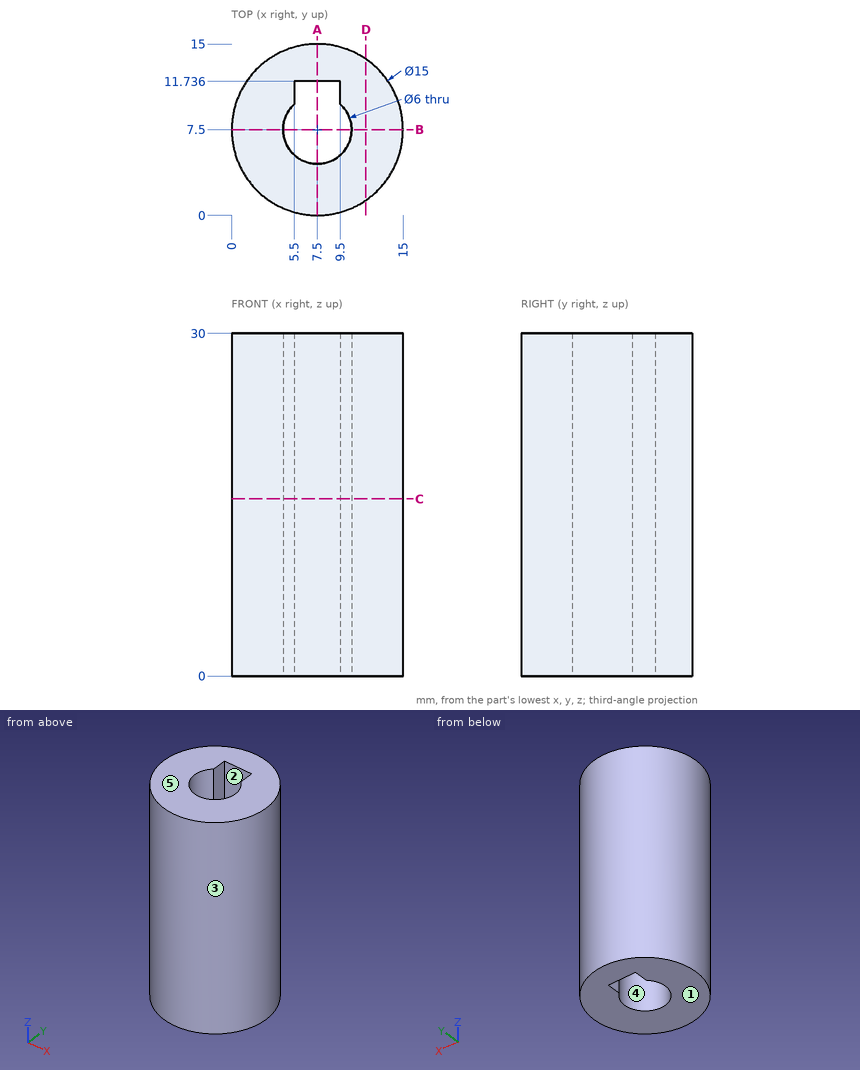
Could you check a few things on this drawing? It's one solid part, dimensions in mm from its lowest x, y, z. A direction names the side the tool comes from. Give positions to 0.01 mm unless a question says otherwise; leave off trailing zeros. Order: outer loops, then holes, each group sorted by start corner. A loop starts at its lowest first (then second) coordinate and runs counter-clockwise, first axis right, second up. Notation, with made-up numbers: (-26, 37) - (13, 37) arc R22 ccw to (13, 46) - close; hole circle Ø11 at (-14.75, 6.5). An arc over 180 degrees is marked (long way). Return JSON: item names as keys, results as strings. Group by question number.
Q1. Thinking about a two-plate mould opening in Y: for the marked faces 3, 4 and 5, which applies, pulls with the +Y half, pulls with the -Y half, needs draft (parallel to the pull), parting line crosses it, or undercut?
Q2. Suppose I cut it at D-D, the plane x = 11.75. Please give me the cut outline in (y, z), and give its area (3 significant figures).
Q3. Suppose I cut it at C-C, the plane z = 15.5. Please give me the cut outline in (x, y), and give its area (3 significant figures).
Q4. Suppose I cut it at B-B, the plane y = 7.5. Please give me the cut outline in (x, z).
Q5. Will these pins go through, and if not, where does the flat tip stop? pin 1 Ø0.6 at (y, z) = (11, 8) entering from -X; pin 2 Ø5 at (y, z) = (13, 10) entering from -X; pin 3 Ø3 at (y, z) = (1.5, 9.5) entering from -X; pin 4 Ø1 at (x, y) = (5.5, 8) entering from +Z.
Q6. Suppose I cut it at A-A, the plane x = 7.5. Please give me the cut outline in (y, z), and give its area (3 significant figures).
Q7. Please list where these lines run through material, in increasing order: line 1 along Y through (x, z) = (7.5, 10); line 2 along X through (y, z) = (10.5, 18); line 3 along X through (y, z) = (6, 26.75). Write a range as [from, to].
Q8. Which directions (+Z, -Z, +X, -X, +Y, -Y) give clear straight access to the entire face, cutting with the end or side of a thin tool? Please do the marked faces 1 and 2.
Resolved:
{
 "1": {"face 3": "parting line crosses it", "face 4": "undercut", "face 5": "needs draft"},
 "2": {"outline": "(1.32, 0) - (13.68, 0) - (13.68, 30) - (1.32, 30) - close", "area": "371 mm2"},
 "3": {"outline": "circle Ø15 at (7.5, 7.5); hole (5.5, 9.74) arc R3 ccw (long way) to (9.5, 9.74) - (9.5, 11.74) - (5.5, 11.74) - close", "area": "143 mm2"},
 "4": {"outline": "(0, 0) - (4.5, 0) - (4.5, 30) - (0, 30) - close; (10.5, 0) - (15, 0) - (15, 30) - (10.5, 30) - close"},
 "5": {"pin 1": "stops at x = 0.72", "pin 2": "stops at x = 0.63", "pin 3": "stops at x = 1.5", "pin 4": "passes through"},
 "6": {"outline": "(0, 0) - (4.5, 0) - (4.5, 30) - (0, 30) - close; (11.74, 0) - (15, 0) - (15, 30) - (11.74, 30) - close", "area": "233 mm2"},
 "7": {"line 1": "y = [0, 4.5], [11.74, 15]", "line 2": "x = [0.63, 5.5], [9.5, 14.37]", "line 3": "x = [0.15, 4.9], [10.1, 14.85]"},
 "8": {"face 1": "-Z, +X, -X, +Y, -Y", "face 2": "+Z, -Z"}
}
